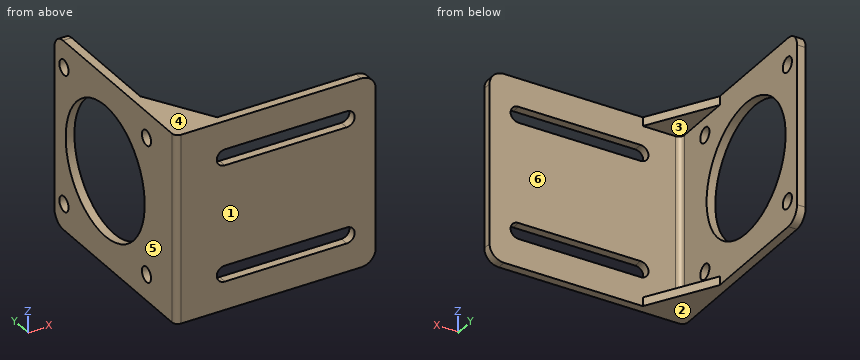
Autodesk Inventor part; units mm, degrees
ref_plane "YZ Plane" through (0, 0, 0) normal (1, 0, 0) x (0, 1, 0)
ref_plane "XZ Plane" through (0, 0, 0) normal (0, 1, 0) x (-1, 0, 0)
ref_plane "XY Plane" through (0, 0, 0) normal (0, 0, 1) x (1, 0, 0)
sketch "Sketch1" plane through (0, 0, 0) normal (0, 1, 0) x (-1, 0, 0)
  line L0 (0, 0) -> (69, 0)
  line L1 (69, 0) -> (69, -65)
  line L2 (69, -65) -> (0, -65)
  line L3 (0, -65) -> (0, 0)
  dimension "d0" = 69
  dimension "d1" = 65
extrude "Extrusion1" add sketch "Sketch1" along normal blind 3
sketch "Sketch2" plane through (0, 3, 0) normal (0, 1, 0) x (1, 0, 0)
  line L0 (0, 65) -> (-69, 65)
  line L1 (-69, 65) -> (-66, 65)
  line L2 (-66, 65) -> (-66, 0)
  line L3 (-66, 0) -> (-69, 0)
  line L4 (-69, 0) -> (-69, 65)
  point P0 (0, 0)
  dimension "d4" = 3
  dimension "d5" = 65
extrude "Extrusion2" add sketch "Sketch2" along normal blind 66
fillet "Fillet1" radius 2 2 edges at (-66, 3, -32.5) (-69, 0, -32.5)
sketch "Sketch3" plane through (0, 0, 0) normal (0, 0, 1) x (1, 0, 0)
  line L0 (-67, 0) -> (0, 0)
  line L1 (-66, 0) -> (-51, 0) construction
  line L2 (-66, 5) -> (-66, 69)
  line L3 (-66, 5) -> (-66, 0)
  line L4 (-66, 5) -> (-61, 5) construction
  line L5 (-66, 0) -> (-51, 0)
  line L6 (-66, 0) -> (-66, 25)
  line L7 (-66, 25) -> (-51, 0)
  dimension "d12" = 5
  dimension "d13" = 90
  dimension "d14" = 15
  dimension "d15" = 90
  dimension "d16" = 25
extrude "Extrusion3" add sketch "Sketch3" against normal blind 3
pattern_linear "Rectangular Pattern1" count 2 spacing 62 along (0, 0, -1) of "Extrusion3"
sketch "Sketch4" plane through (-66, 69, 0) normal (1, 0, 0) x (0, 0, -1)
  circle A0 centre (32.5, -29) radius 22.5
  line L0 (0, 0) -> (65, 0)
  line L1 (0, -44) -> (0, 0)
  point P0 (0, -69)
  dimension "d22" = 45
  dimension "d23" = 29
  dimension "d24" = 32.5
extrude "Extrusion4" cut sketch "Sketch4" against normal blind 3
sketch "Sketch5" plane through (-66, 69, 0) normal (1, 0, 0) x (0, 0, -1)
  circle A0 centre (9, -5.501) radius 2.6
  line L0 (0, 0) -> (65, 0)
  line L1 (0, -44) -> (0, 0)
  circle A1 centre (56, -5.501) radius 2.6
  circle A2 centre (9, -52.501) radius 2.6
  circle A3 centre (56, -52.501) radius 2.6
  point P0 (0, -69)
  dimension "d27" = 5.2
  dimension "d28" = 5.501
  dimension "d29" = 9
  dimension "d32" = 47
  dimension "d35" = 47
extrude "Extrusion5" cut sketch "Sketch5" against normal blind 3
sketch "Sketch6" plane through (0, 3, 0) normal (0, 1, 0) x (1, 0, 0)
  line L0 (-52.8, 0) -> (0, 0)
  line L1 (0, 0) -> (0, 65)
  arc A0 (-51.9673, 15.2498) -> (-52, 9.75) centre (-52, 12.5) ccw
  line L2 (-69, 65) -> (-69, 0)
  line L3 (-11.5517, 12.5) -> (-9.4517, 12.5) construction
  line L4 (-11.5517, 9.75) -> (-52, 9.75)
  line L5 (-52, 12.5) -> (-10, 12.5) construction
  line L6 (-52, 9.75) -> (-10, 9.75)
  line L7 (-10, 15.25) -> (-52, 15.25)
  arc A1 (-52, 15.25) -> (-52, 9.75) centre (-52, 12.5) ccw
  arc A2 (-10, 9.75) -> (-10, 15.25) centre (-10, 12.5) ccw
  point P0 (-31, 12.5)
  dimension "d48" = 5.5
  dimension "d49" = 12.5
  dimension "d50" = 12.5
  dimension "d54" = 17
  dimension "d62" = 42
  dimension "d63" = 5.5
extrude "Extrusion6" cut sketch "Sketch6" against normal blind 3
pattern_linear "Rectangular Pattern2" count 2 spacing 40 along (0, 0, -1) of "Extrusion6"
fillet "Fillet2" radius 5 2 edges at (-67.5, 69, 0) (-67.5, 69, -65)
fillet "Fillet3" radius 5 2 edges at (0, 1.5, 0) (0, 1.5, -65)
properties part number "NEMA23_StepperonlineMount"
Here's how the part is built. I have some questions about the finished solid (model axes, mm). Face numbers are marked on the shaded views. A direction names the side the tool comes from. Coordinates: 2 decimals unless noted, no trailing zeros. Write each loop counter-clockwise with the first axis right and the second up, starting at its lowest first coordinate (ties: lowest second). Pieces come first, ordered by that corner, then holes. Notation, with made-up numbers: (-6.5, -3) -> (18.5, -3) arc R34 ccw to (18.5, 36) -> close; hole circle Ø6 at (-30.75, -6). An arc over 180 degrees is marked (long way). Use a Markdown table: item, result. Add a question column.
(1) If we section it at D-D, the plane x = -61.5: Write out the boundary of the cut face in (y, z).
(2) If we section it at A-A, the plane x = -25.5: Write out the boundary of the cut face in (y, z).
(3) For the marked faces 5 and 6, which set-ups out of +Z, -Z, +X, -X, +Y, -Y let a thin tool reach every point of the face, with its end or its side?
(4) If we section it at B-B, the plane y = 40: Write out the boundary of the cut face in (x, z), and give its area (3 significant figures).
(5) I'm going to push a flat-ended pin straight in: P1, Ø19, axis at x = -36, z = -18, coming from the +Y side. Where does the tip first touch, or does it pass through?
(6) Please list where these lines run through material, in increasing order: line 1 (Y direction, x = -67.25, z = -56); line 2 (Y direction, x = -67.7, z = -56); line 3 (Z direction, x = -55.5, y = 4.5).
(7) We'd pull the mould along Z, two halves only. Please class the marked faces 1, 2, 3 and 4: +Z half, -Z half, draft (parallel to the pull), parting line (faces both ways), or undercut.
(8) If we section it at C-C, the plane z = -32.5: Write out the boundary of the cut face in (x, y), and give its area (3 significant figures).
Outcome:
| question | item | result |
|---|---|---|
| 1 | outline | (0, -65) -> (17.5, -65) -> (17.5, -62) -> (3, -62) -> (3, -3) -> (17.5, -3) -> (17.5, 0) -> (0, 0) -> close |
| 2 | outline | (0, -65) -> (3, -65) -> (3, -55.25) -> (0, -55.25) -> close; (0, -49.75) -> (3, -49.75) -> (3, -15.25) -> (0, -15.25) -> close; (0, -9.75) -> (3, -9.75) -> (3, 0) -> (0, 0) -> close |
| 3 | face 5 | +Z, -Z, -X, +Y, -Y |
| 3 | face 6 | +X, +Y |
| 4 | outline | (-69, -65) -> (-66, -65) -> (-66, -55) -> (-69, -55) -> close; (-69, -10) -> (-66, -10) -> (-66, 0) -> (-69, 0) -> close |
| 4 | area | 60.0 mm^2 |
| 5 | P1 | stops at y = 3 |
| 6 | line 1 | y = 0.02 to 13.9, 19.1 to 60.9, 66.1 to 69 |
| 6 | line 2 | y = 0.13 to 13.9, 19.1 to 60.9, 66.1 to 69 |
| 6 | line 3 | z = -65 to -62, -3 to 0 |
| 7 | face 1 | draft |
| 7 | face 2 | -Z half |
| 7 | face 3 | undercut |
| 7 | face 4 | +Z half |
| 8 | outline | (-69, 2) arc R2 ccw to (-67, 0) -> (0, 0) -> (0, 3) -> (-64, 3) arc R2 cw to (-66, 5) -> (-66, 17.5) -> (-69, 17.5) -> close; (-69, 62.5) -> (-66, 62.5) -> (-66, 69) -> (-69, 69) -> close |
| 8 | area | 270 mm^2 |
